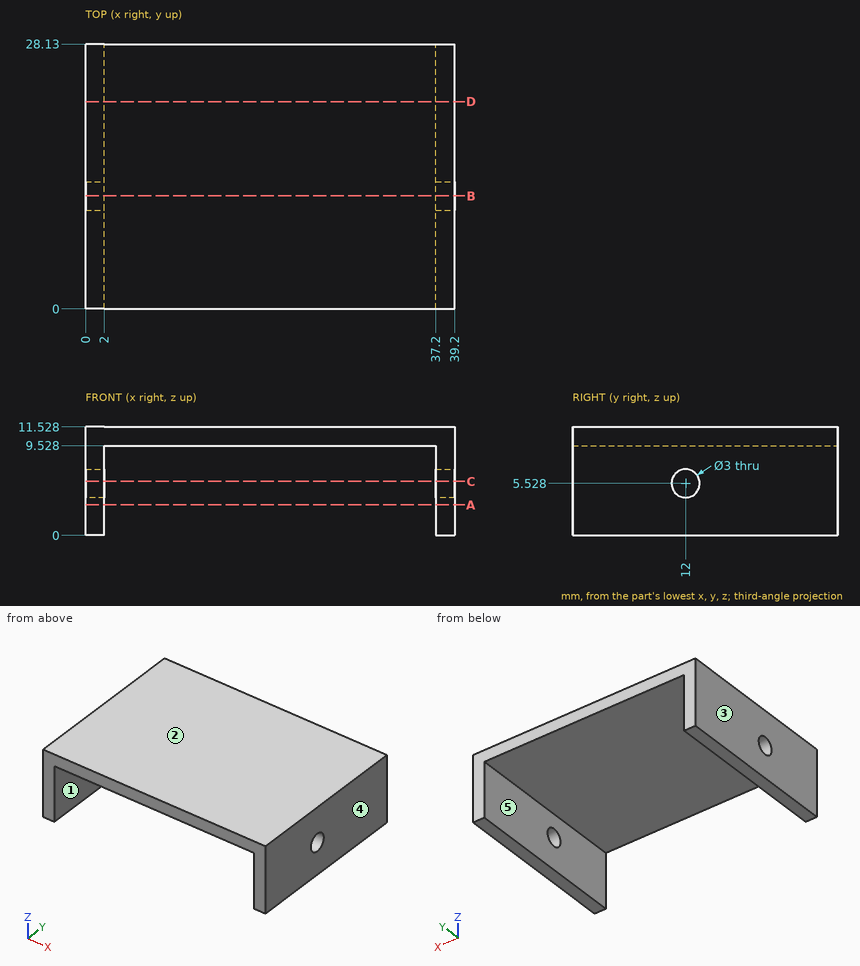
Study the drawing (mm; zero at the part's minimum x, y, z) and answer. A direction names the side the tool comes from. Round coordinates to 2 decimals unless told otherwise and drop trailing zeros. Write each loop counter-clockwise with the first axis right and the second up, starting at its lowest first coordinate (ties: lowest second). Pieces come first, ordered by that corner, then holes. Notation, with made-up numbers: (1.5, -31.75) - (56.5, -31.75) arc R29 cw to (56.5, -9.75) - close; hole circle Ø7 at (74.25, 5.5). An arc over 180 degrees is marked (long way). Return JSON: item names as keys, results as strings. Group by question number.
Q1. Find the intervals of material crossed by L1, parallel to X at y = 8.75, z = 5.5; L2, parallel to Z at x = 8.5, y = 15.5, in increasing order.
Q2. For the marked faces 1 and 2, determine the directions among +Z, -Z, +X, -X, +Y, -Y from which every point of the face is accessible in a straight line to the end or side of a thin tool.
Q3. The mould has two halves that part along X. Classify the marked faces 3, 4 and 5: released by +X, released by -X, zero draft, split by the parting line, or undercut.
Q4. The part is cut by section D-D on y = 22. Write down the section's boundary in (x, z).
Q5. The part is cut by section C-C on z = 5.75. Write down the section's boundary in (x, y), then the cut area to 3 significant figures.
Q6. The part is cut by section B-B on y = 12. Write down the section's boundary in (x, z).
Q7. Each of these flat-tipped pins is pushed along its axis until it touches: pin 1 Ø4 at (y, z) = (12, 5.53) entering from +X; pin 2 Ø12 at (x, y) = (23.5, 18) entering from -Z. Where does it stop, or does it pass through?
Q8. The part is cut by section A-A on z = 3.25. Write down the section's boundary in (x, y).
Solved:
{
 "1": {"L1": "0 to 2, 37.2 to 39.2", "L2": "9.53 to 11.53"},
 "2": {"face 1": "-Z, +Y, -Y", "face 2": "+Z, +X, -X, +Y, -Y"},
 "3": {"face 3": "released by -X", "face 4": "released by +X", "face 5": "undercut"},
 "4": {"outline": "(0, 0) - (2, 0) - (2, 9.53) - (37.2, 9.53) - (37.2, 0) - (39.2, 0) - (39.2, 11.53) - (0, 11.53) - close"},
 "5": {"outline": "(0, 0) - (2, 0) - (2, 10.52) - (0, 10.52) - close; (0, 13.48) - (2, 13.48) - (2, 28.13) - (0, 28.13) - close; (37.2, 0) - (39.2, 0) - (39.2, 10.52) - (37.2, 10.52) - close; (37.2, 13.48) - (39.2, 13.48) - (39.2, 28.13) - (37.2, 28.13) - close", "area": "101 mm²"},
 "6": {"outline": "(0, 0) - (2, 0) - (2, 4.03) - (0, 4.03) - close; (0, 7.03) - (2, 7.03) - (2, 9.53) - (37.2, 9.53) - (37.2, 7.03) - (39.2, 7.03) - (39.2, 11.53) - (0, 11.53) - close; (37.2, 0) - (39.2, 0) - (39.2, 4.03) - (37.2, 4.03) - close"},
 "7": {"pin 1": "x = 39.2", "pin 2": "z = 9.53"},
 "8": {"outline": "(0, 0) - (2, 0) - (2, 28.13) - (0, 28.13) - close; (37.2, 0) - (39.2, 0) - (39.2, 28.13) - (37.2, 28.13) - close"}
}
